Part print with two shaded views. Sizes in mm from the minimum x, y, z corner. A direction names the side the tool comes from. Give positions to 0.01 mm unless a question says otherwise; leave off trailing zeros. Loops run counter-clockwise (first coordinate to the right, second up) from the corner with the lowest first, then second, coordinate; pieces in that order, holes last. Notation, with made-up numbers: M 16.5,20 L 69.5,20 A21 cw 69.5,56 Z; hole C 44.5,-29.75 d2. An arc over 180 degrees is marked long. Answer in a Markdown table with one row per item.
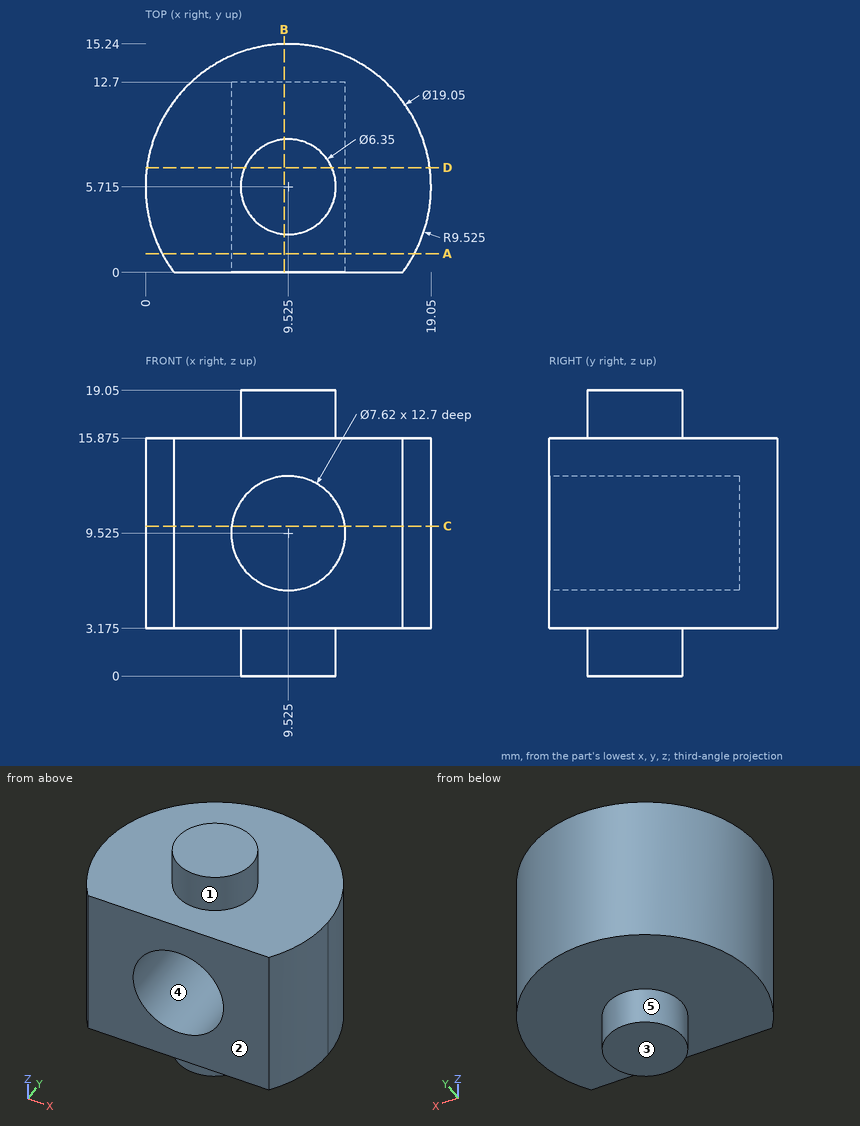
Q1. Probe probe 1 along Z at (x, y) = (17.5, 4) (3 decimals); probe 2 along Z at (x, y) = (11, 10) (3 decimals); probe 3 along Z at (x, y) = (9.5, 4). List the from-to ranges inside material, lowest first.
Reported:
| item | result |
|---|---|
| probe 1 | 3.175 to 15.875 |
| probe 2 | 3.175 to 6.012, 13.038 to 15.875 |
| probe 3 | 0 to 5.72, 13.33 to 19.05 |
Q2. Saw through at A-A (y = 1.25). Give the cut face in (x, z) (3 decimals).
Reported:
| item | result |
|---|---|
| outline | M 1.111,3.175 L 17.939,3.175 L 17.939,15.875 L 1.111,15.875 Z; hole C 9.525,9.525 d7.62 |
Q3. Saw through at C-C (z = 10). Give the cut face in (x, y) (3 decimals).
Reported:
| item | result |
|---|---|
| outline | M 1.905,0 L 5.745,0 L 5.745,12.7 L 13.305,12.7 L 13.305,0 L 17.145,0 A9.525 ccw long Z |
Q4. Saw through at D-D (y = 7). Give the cut face in (x, z) (3 decimals).
Reported:
| item | result |
|---|---|
| outline | M 0.087,3.175 L 6.622,3.175 L 6.622,0 L 12.428,0 L 12.428,3.175 L 18.963,3.175 L 18.963,15.875 L 12.428,15.875 L 12.428,19.05 L 6.622,19.05 L 6.622,15.875 L 0.087,15.875 Z; hole C 9.525,9.525 d7.62 |
Q5. Saw through at B-B (x = 9.25). Give the cut face in (y, z) (3 decimals).
Reported:
| item | result |
|---|---|
| outline | M 0,3.175 L 2.552,3.175 L 2.552,0 L 8.878,0 L 8.878,3.175 L 15.236,3.175 L 15.236,15.875 L 8.878,15.875 L 8.878,19.05 L 2.552,19.05 L 2.552,15.875 L 0,15.875 L 0,13.325 L 12.7,13.325 L 12.7,5.725 L 0,5.725 Z |
Q6. 3-axis set-ups, long thin cutter, end or side, ignore diameter. For the marked faces 1 and 2: which of +Z, -Z, +X, -X, +Y, -Y reach the whole face in a straight line?
Reported:
| item | result |
|---|---|
| face 1 | +Z |
| face 2 | +Z, -Z, +X, -X, -Y |
Q7. Drop flat-ended pins along their axis: pin 1 (4 mm diameter, centred on y = 2, z = 15.5, fed in from +X); pin 2 (4.5 mm diameter, centred on x = 8, y = 10, fed in from +Z); pin 3 (7 mm diameter, centred on x = 9.525, z = 9.525, fed in from -Y); pin 4 (2 mm diameter, centred on y = 1.5, z = 9, fed in from -X). Give the stop position or say it passes through.
Reported:
| item | result |
|---|---|
| pin 1 | x = 18.89 |
| pin 2 | z = 19.05 |
| pin 3 | y = 12.7 |
| pin 4 | x = 0.56 |
Q8. Mould opens along Z. For the marked faces 3, 4 and 5 say: released by +Z, released by -Z, zero draft, split by the parting line, or undercut.
Reported:
| item | result |
|---|---|
| face 3 | released by -Z |
| face 4 | undercut |
| face 5 | zero draft |
